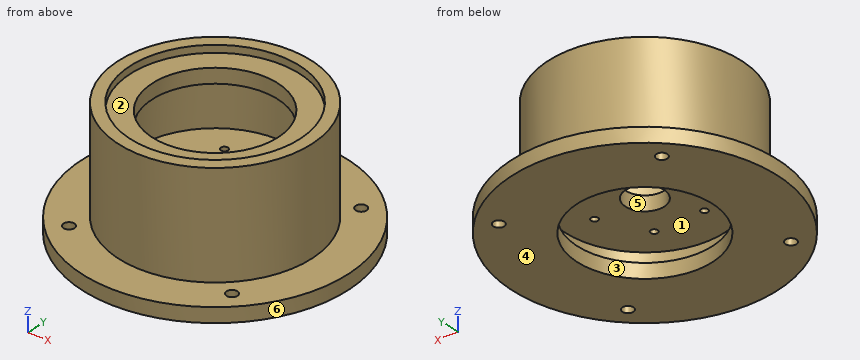
from build123d import *

# Parameters (mm, degrees)
BRIDA_START                               = 10
SK_BRIDA_R                                = 55
BRIDA_DEPTH                               = 6
TUBO_START                                = 16
SK_TUBO_R                                 = 40
SK_TUBO_R_2                               = 33
TUBO_DEPTH                                = 34
ARO_RODAMIENTO_START                      = 50
SK_ARO_RODAMIENTO_R                       = 40
SK_ARO_RODAMIENTO_R_2                     = 26
ARO_RODAMIENTO_DEPTH                      = 6
ASIENTO_ARANDELA_ALOJAMIENTO_51110_START  = 56
SK_ASIENTO_ARANDELA_ALOJAMIENTO_51110_R   = 40
SK_ASIENTO_ARANDELA_ALOJAMIENTO_51110_R_2 = 35.1
ASIENTO_ARANDELA_ALOJAMIENTO_51110_DEPTH  = 3
PLACA_MOTOR_START                         = 23
SK_PLACA_MOTOR_R                          = 33
PLACA_MOTOR_DEPTH                         = 6
HUECO_BRIDA_START                         = 10
SK_HUECO_BRIDA_R                          = 28
HUECO_BRIDA_DEPTH                         = 13
CENTRO_MOTOR_START                        = 23
SK_CENTRO_MOTOR_R                         = 8
CENTRO_MOTOR_DEPTH                        = 6
PASANTES_M2_5_MOTOR_START                 = 23
SK_PASANTES_M2_5_MOTOR_R                  = 1.45
PASANTES_M2_5_MOTOR_DEPTH                 = 6
PASANTES_M4_BRIDA_START                   = 10
SK_PASANTES_M4_BRIDA_R                    = 2.25
PASANTES_M4_BRIDA_DEPTH                   = 6


with BuildPart() as part:
    # Sk_Brida → Brida (new body)
    with BuildSketch(Plane.XY.offset(BRIDA_START)):
        Circle(SK_BRIDA_R)
    extrude(amount=BRIDA_DEPTH)

    # Sk_Tubo → Tubo (add)
    with BuildSketch(Plane.XY.offset(TUBO_START)):
        Circle(SK_TUBO_R)
        Circle(SK_TUBO_R_2, mode=Mode.SUBTRACT)
    extrude(amount=TUBO_DEPTH)

    # Sk_Aro_rodamiento → Aro_rodamiento (add)
    with BuildSketch(Plane.XY.offset(ARO_RODAMIENTO_START)):
        Circle(SK_ARO_RODAMIENTO_R)
        Circle(SK_ARO_RODAMIENTO_R_2, mode=Mode.SUBTRACT)
    extrude(amount=ARO_RODAMIENTO_DEPTH)

    # Sk_Asiento_arandela_alojamiento_51110 → Asiento_arandela_alojamiento_51110 (add)
    with BuildSketch(Plane.XY.offset(ASIENTO_ARANDELA_ALOJAMIENTO_51110_START)):
        Circle(SK_ASIENTO_ARANDELA_ALOJAMIENTO_51110_R)
        Circle(SK_ASIENTO_ARANDELA_ALOJAMIENTO_51110_R_2, mode=Mode.SUBTRACT)
    extrude(amount=ASIENTO_ARANDELA_ALOJAMIENTO_51110_DEPTH)

    # Sk_Placa_motor → Placa_motor (add)
    with BuildSketch(Plane.XY.offset(PLACA_MOTOR_START)):
        Circle(SK_PLACA_MOTOR_R)
    extrude(amount=PLACA_MOTOR_DEPTH)

    # Sk_Hueco_brida → Hueco_brida (cut)
    with BuildSketch(Plane.XY.offset(HUECO_BRIDA_START)):
        Circle(SK_HUECO_BRIDA_R)
    extrude(amount=HUECO_BRIDA_DEPTH, mode=Mode.SUBTRACT)

    # Sk_Centro_motor → Centro_motor (cut)
    with BuildSketch(Plane.XY.offset(CENTRO_MOTOR_START)):
        Circle(SK_CENTRO_MOTOR_R)
    extrude(amount=CENTRO_MOTOR_DEPTH, mode=Mode.SUBTRACT)

    # Sk_Pasantes_M2-5_motor → Pasantes_M2-5_motor (cut)
    with BuildSketch(Plane.XY.offset(PASANTES_M2_5_MOTOR_START)):
        with Locations((20.5, 0)):
            Circle(SK_PASANTES_M2_5_MOTOR_R)
        with Locations((10.25, 17.753520778)):
            Circle(SK_PASANTES_M2_5_MOTOR_R)
        with Locations((-10.25, 17.753520778)):
            Circle(SK_PASANTES_M2_5_MOTOR_R)
        with Locations((-20.5, 0)):
            Circle(SK_PASANTES_M2_5_MOTOR_R)
        with Locations((-10.25, -17.753520778)):
            Circle(SK_PASANTES_M2_5_MOTOR_R)
        with Locations((10.25, -17.753520778)):
            Circle(SK_PASANTES_M2_5_MOTOR_R)
    extrude(amount=PASANTES_M2_5_MOTOR_DEPTH, mode=Mode.SUBTRACT)

    # Sk_Pasantes_M4_brida → Pasantes_M4_brida (cut)
    with BuildSketch(Plane.XY.offset(PASANTES_M4_BRIDA_START)):
        with Locations((33.234018716, 33.234018716)):
            Circle(SK_PASANTES_M4_BRIDA_R)
        with Locations((-33.234018716, 33.234018716)):
            Circle(SK_PASANTES_M4_BRIDA_R)
        with Locations((-33.234018716, -33.234018716)):
            Circle(SK_PASANTES_M4_BRIDA_R)
        with Locations((33.234018716, -33.234018716)):
            Circle(SK_PASANTES_M4_BRIDA_R)
    extrude(amount=PASANTES_M4_BRIDA_DEPTH, mode=Mode.SUBTRACT)


solid = part.part
Geometry check sheet. Reference: the model listing, model coordinates, mm. Face numbers are marked on the shaded views. A direction names the side the tool comes from. Give positions to 0.01 mm unless a question says otherwise; leave off trailing zeros. Order: outer loops, then holes, each group sorted by start corner. A loop starts at its lowest first (then second) coordinate and runs counter-clockwise, first axis right, second up. Notation, with made-up numbers: M 68.25,53 L 102.25,53 A25 ccw 102.25,86 Z; hole C 87,33.5 d1. An arc over 180 degrees is marked long. Use a Markdown table: item, result.
Item 1: Tool access check on the marked faces 1, 2 and 3. Record the directions out of +Z, -Z, +X, -X, +Y, -Y that give a thin tool (end or side, any length) a straight path to the whole face; none if there is none.
Answers follow:
| item | result |
|---|---|
| face 1 | none |
| face 2 | +Z |
| face 3 | -Z |
Item 2: Section check D-D (z = 42). Record the cut outline in (x, y), and give its area (3 significant figures).
Answers follow:
| item | result |
|---|---|
| outline | C 0,0 d80; hole C 0,0 d66 |
| area | 1,610 mm2 |
Item 3: Section check C-C (x = 37). Record the cut outline in (y, z), and give its area (3 significant figures).
Answers follow:
| item | result |
|---|---|
| outline | M -40.69,10 L 40.69,10 L 40.69,16 L 15.2,16 L 15.2,59 L -15.2,59 L -15.2,16 L -40.69,16 Z |
| area | 1,800 mm2 |
Item 4: Draft check along Y on the marked faces 4, 5 and 6. Enter one of: +Y half, -Y half, draft (parallel to the pull), parting line (faces both ways), or undercut.
Answers follow:
| item | result |
|---|---|
| face 4 | draft |
| face 5 | undercut |
| face 6 | parting line |
Item 5: Depth check by flat-ended pin: P1, Ø3.5, axis at x = -33.23, y = 33.23, coming from the -Z side; P2, Ø10, axis at x = -32, z = 29.5, coming from the +Y side; P3, Ø4, axis at x = -20.5, y = 0, coming from the +Z side; P4, Ø1, axis at y = 37, z = 16, coming from the -X side. Enter the tip coordinate at first touch or a pass-through.
Answers follow:
| item | result |
|---|---|
| P1 | passes through |
| P2 | stops at y = 29.51 |
| P3 | stops at z = 29 |
| P4 | stops at x = -41.14 |
Item 6: Material ranges on line 1 along Y through (x, z) = (0, 27.15); line 2 along Y through (x, z) = (10, 26); line 3 along Z through (x, y) = (0, -26.5), recorded low to high.
Answers follow:
| item | result |
|---|---|
| line 1 | y = -40 to -8, 8 to 40 |
| line 2 | y = -38.73 to -19.18, -16.33 to 16.33, 19.18 to 38.73 |
| line 3 | z = 23 to 29, 50 to 56 |
